Design review of the part built by this model. Coordinates are the model's own, in mm. Give positions to 0.01 mm unless a question says otherwise; leave off trailing zeros. Write each loop counter-clockwise with the first axis right and the second up, starting at its lowest first coordinate (ties: lowest second). Pieces come first, ordered by that corner, then holes. Notation, with made-up numbers: (79.5, -23) -> (111.5, -23) arc R21 cw to (111.5, -16) -> close; hole circle Ø8 at (8.25, 52). An arc over 180 degrees is marked (long way). Return JSON: item names as keys, results as strings. Group by question number.
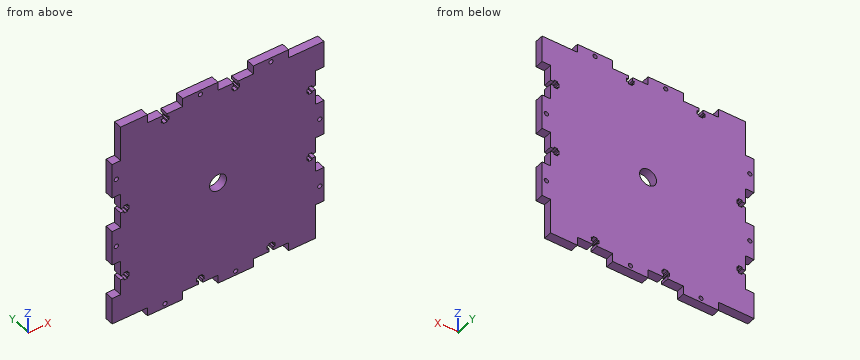
from build123d import *

# Parameters (mm, degrees)
BOSS_EXTRUDE1_DEPTH = 6
SKETCH2_R           = 1.5
CUT_EXTRUDE1_DEPTH  = 107.235587258
SKETCH3_R           = 6
CUT_EXTRUDE2_DEPTH  = 107.235587258


with BuildPart() as part:
    # Sketch1 → Boss-Extrude1 (new body)
    with BuildSketch(Plane(origin=(0, 0, 0), x_dir=(1, 0, 0), z_dir=(0, 1, 0))):
        Polygon((0, 75), (25, 75), (25, 69), (50, 69), (50, 75), (69, 75), (69, 50), (75, 50), (75, 25), (69, 25), (69, 0), (75, 0), (75, -25), (69, -25), (69, -50), (75, -50), (75, -69), (50, -69), (50, -75), (25, -75), (25, -69), (0, -69), (0, -75), (-25, -75), (-25, -69), (-50, -69), (-50, -75), (-69, -75), (-69, -50), (-75, -50), (-75, -25), (-69, -25), (-69, 0), (-75, 0), (-75, 25), (-69, 25), (-69, 50), (-75, 50), (-75, 69), (-50, 69), (-50, 75), (-25, 75), (-25, 69), (0, 69), align=None)
    extrude(amount=BOSS_EXTRUDE1_DEPTH)

    # Sketch2 → Cut-Extrude1 (cut, through all)
    with BuildSketch(Plane(origin=(0, 6, 0), x_dir=(1, 0, 0), z_dir=(0, 1, 0))):
        with Locations(Location((-37.5, 72, 0), (0, 0, 270))):
            Circle(SKETCH2_R)
        with Locations(Location((12.5, 72, 0), (0, 0, 270))):
            Circle(SKETCH2_R)
        with Locations(Location((72, 37.5, 0), (0, 0, 270))):
            Circle(SKETCH2_R)
        with Locations(Location((72, -12.5, 0), (0, 0, 270))):
            Circle(SKETCH2_R)
        with Locations(Location((37.5, -72, 0), (0, 0, 270))):
            Circle(SKETCH2_R)
        with Locations(Location((-12.5, -72, 0), (0, 0, 270))):
            Circle(SKETCH2_R)
        with Locations(Location((-72, -37.5, 0), (0, 0, 270))):
            Circle(SKETCH2_R)
        with Locations(Location((-72, 12.5, 0), (0, 0, 270))):
            Circle(SKETCH2_R)
        with BuildLine():
            Line((-11, 69), (-14, 69))
            Line((-14, 69), (-14, 66.6))
            Line((-14, 66.6), (-15.1, 66.6))
            ThreePointArc((-15.1, 66.6), (-15.270710678, 66.670710678), (-15.2, 66.5))
            Line((-15.2, 66.5), (-15.2, 64.3))
            ThreePointArc((-15.2, 64.3), (-15.270710678, 64.129289322), (-15.1, 64.2))
            Line((-15.1, 64.2), (-14, 64.2))
            Line((-14, 64.2), (-14, 63))
            Line((-14, 63), (-11, 63))
            Line((-11, 63), (-11, 64.2))
            Line((-11, 64.2), (-9.9, 64.2))
            ThreePointArc((-9.9, 64.2), (-9.729289322, 64.129289322), (-9.8, 64.3))
            Line((-9.8, 64.3), (-9.8, 66.5))
            ThreePointArc((-9.8, 66.5), (-9.729289322, 66.670710678), (-9.9, 66.6))
            Line((-9.9, 66.6), (-11, 66.6))
            Line((-11, 66.6), (-11, 69))
        make_face()
        with BuildLine():
            Line((69, 11), (69, 14))
            Line((69, 14), (66.6, 14))
            Line((66.6, 14), (66.6, 15.1))
            ThreePointArc((66.6, 15.1), (66.670710678, 15.270710678), (66.5, 15.2))
            Line((66.5, 15.2), (64.3, 15.2))
            ThreePointArc((64.3, 15.2), (64.129289322, 15.270710678), (64.2, 15.1))
            Line((64.2, 15.1), (64.2, 14))
            Line((64.2, 14), (63, 14))
            Line((63, 14), (63, 11))
            Line((63, 11), (64.2, 11))
            Line((64.2, 11), (64.2, 9.9))
            ThreePointArc((64.2, 9.9), (64.129289322, 9.729289322), (64.3, 9.8))
            Line((64.3, 9.8), (66.5, 9.8))
            ThreePointArc((66.5, 9.8), (66.670710678, 9.729289322), (66.6, 9.9))
            Line((66.6, 9.9), (66.6, 11))
            Line((66.6, 11), (69, 11))
        make_face()
        with BuildLine():
            Line((39, 69), (36, 69))
            Line((36, 69), (36, 66.6))
            Line((36, 66.6), (34.9, 66.6))
            ThreePointArc((34.9, 66.6), (34.729289322, 66.670710678), (34.8, 66.5))
            Line((34.8, 66.5), (34.8, 64.3))
            ThreePointArc((34.8, 64.3), (34.729289322, 64.129289322), (34.9, 64.2))
            Line((34.9, 64.2), (36, 64.2))
            Line((36, 64.2), (36, 63))
            Line((36, 63), (39, 63))
            Line((39, 63), (39, 64.2))
            Line((39, 64.2), (40.1, 64.2))
            ThreePointArc((40.1, 64.2), (40.270710678, 64.129289322), (40.2, 64.3))
            Line((40.2, 64.3), (40.2, 66.5))
            ThreePointArc((40.2, 66.5), (40.270710678, 66.670710678), (40.1, 66.6))
            Line((40.1, 66.6), (39, 66.6))
            Line((39, 66.6), (39, 69))
        make_face()
        with BuildLine():
            Line((69, -39), (69, -36))
            Line((69, -36), (66.6, -36))
            Line((66.6, -36), (66.6, -34.9))
            ThreePointArc((66.6, -34.9), (66.670710678, -34.729289322), (66.5, -34.8))
            Line((66.5, -34.8), (64.3, -34.8))
            ThreePointArc((64.3, -34.8), (64.129289322, -34.729289322), (64.2, -34.9))
            Line((64.2, -34.9), (64.2, -36))
            Line((64.2, -36), (63, -36))
            Line((63, -36), (63, -39))
            Line((63, -39), (64.2, -39))
            Line((64.2, -39), (64.2, -40.1))
            ThreePointArc((64.2, -40.1), (64.129289322, -40.270710678), (64.3, -40.2))
            Line((64.3, -40.2), (66.5, -40.2))
            ThreePointArc((66.5, -40.2), (66.670710678, -40.270710678), (66.6, -40.1))
            Line((66.6, -40.1), (66.6, -39))
            Line((66.6, -39), (69, -39))
        make_face()
        with BuildLine():
            Line((11, -69), (14, -69))
            Line((14, -69), (14, -66.6))
            Line((14, -66.6), (15.1, -66.6))
            ThreePointArc((15.1, -66.6), (15.270710678, -66.670710678), (15.2, -66.5))
            Line((15.2, -66.5), (15.2, -64.3))
            ThreePointArc((15.2, -64.3), (15.270710678, -64.129289322), (15.1, -64.2))
            Line((15.1, -64.2), (14, -64.2))
            Line((14, -64.2), (14, -63))
            Line((14, -63), (11, -63))
            Line((11, -63), (11, -64.2))
            Line((11, -64.2), (9.9, -64.2))
            ThreePointArc((9.9, -64.2), (9.729289322, -64.129289322), (9.8, -64.3))
            Line((9.8, -64.3), (9.8, -66.5))
            ThreePointArc((9.8, -66.5), (9.729289322, -66.670710678), (9.9, -66.6))
            Line((9.9, -66.6), (11, -66.6))
            Line((11, -66.6), (11, -69))
        make_face()
        with BuildLine():
            Line((-39, -69), (-36, -69))
            Line((-36, -69), (-36, -66.6))
            Line((-36, -66.6), (-34.9, -66.6))
            ThreePointArc((-34.9, -66.6), (-34.729289322, -66.670710678), (-34.8, -66.5))
            Line((-34.8, -66.5), (-34.8, -64.3))
            ThreePointArc((-34.8, -64.3), (-34.729289322, -64.129289322), (-34.9, -64.2))
            Line((-34.9, -64.2), (-36, -64.2))
            Line((-36, -64.2), (-36, -63))
            Line((-36, -63), (-39, -63))
            Line((-39, -63), (-39, -64.2))
            Line((-39, -64.2), (-40.1, -64.2))
            ThreePointArc((-40.1, -64.2), (-40.270710678, -64.129289322), (-40.2, -64.3))
            Line((-40.2, -64.3), (-40.2, -66.5))
            ThreePointArc((-40.2, -66.5), (-40.270710678, -66.670710678), (-40.1, -66.6))
            Line((-40.1, -66.6), (-39, -66.6))
            Line((-39, -66.6), (-39, -69))
        make_face()
        with BuildLine():
            Line((-69, 39), (-69, 36))
            Line((-69, 36), (-66.6, 36))
            Line((-66.6, 36), (-66.6, 34.9))
            ThreePointArc((-66.6, 34.9), (-66.670710678, 34.729289322), (-66.5, 34.8))
            Line((-66.5, 34.8), (-64.3, 34.8))
            ThreePointArc((-64.3, 34.8), (-64.129289322, 34.729289322), (-64.2, 34.9))
            Line((-64.2, 34.9), (-64.2, 36))
            Line((-64.2, 36), (-63, 36))
            Line((-63, 36), (-63, 39))
            Line((-63, 39), (-64.2, 39))
            Line((-64.2, 39), (-64.2, 40.1))
            ThreePointArc((-64.2, 40.1), (-64.129289322, 40.270710678), (-64.3, 40.2))
            Line((-64.3, 40.2), (-66.5, 40.2))
            ThreePointArc((-66.5, 40.2), (-66.670710678, 40.270710678), (-66.6, 40.1))
            Line((-66.6, 40.1), (-66.6, 39))
            Line((-66.6, 39), (-69, 39))
        make_face()
        with BuildLine():
            Line((-69, -11), (-69, -14))
            Line((-69, -14), (-66.6, -14))
            Line((-66.6, -14), (-66.6, -15.1))
            ThreePointArc((-66.6, -15.1), (-66.670710678, -15.270710678), (-66.5, -15.2))
            Line((-66.5, -15.2), (-64.3, -15.2))
            ThreePointArc((-64.3, -15.2), (-64.129289322, -15.270710678), (-64.2, -15.1))
            Line((-64.2, -15.1), (-64.2, -14))
            Line((-64.2, -14), (-63, -14))
            Line((-63, -14), (-63, -11))
            Line((-63, -11), (-64.2, -11))
            Line((-64.2, -11), (-64.2, -9.9))
            ThreePointArc((-64.2, -9.9), (-64.129289322, -9.729289322), (-64.3, -9.8))
            Line((-64.3, -9.8), (-66.5, -9.8))
            ThreePointArc((-66.5, -9.8), (-66.670710678, -9.729289322), (-66.6, -9.9))
            Line((-66.6, -9.9), (-66.6, -11))
            Line((-66.6, -11), (-69, -11))
        make_face()
    extrude(amount=-CUT_EXTRUDE1_DEPTH, mode=Mode.SUBTRACT)

    # Sketch3 → Cut-Extrude2 (cut, through all)
    with BuildSketch(Plane.XZ):
        with Locations(Location((0, 0, 0), (0, 0, 270))):
            Circle(SKETCH3_R)
    extrude(amount=-CUT_EXTRUDE2_DEPTH, mode=Mode.SUBTRACT)


solid = part.part
Q1. For L1, parallel to Z at x = 68, y = 2.4; L2, parallel to Z at x = 72, y = 2.4; L3, parallel to Z at x = -72, y = 2.1, list the stretches that pass through material, from the lowest coordinate up. Write a range as from..to.
Q2. Take a section at B-B, the plane y = 4.85. Count the separate pieces of the cut face and the enclosed holes in it, plus the area to 3 significant figures.
Q3. Insertion check: pin 1 (0.9 mm diameter, centred on x = 14.5, y = 3.5, fed in from +Z); pin 2 (0.6 mm diameter, centred on y = 3.5, z = 35.5, fed in from +X); pin 3 (0.6 mm diameter, centred on y = 3.5, z = -39.5, fed in from -X). Each pin has a flat end and moves straight along its axis. Give the tip position at first contact, or say it passes through.
Q4. Take a section at A-A, the plane z = -19. Give the boundary of the cut face in (x, y).
Q5. Take a section at C-C, the plane x = -8. Give the boundary of the cut face in (y, z).
Final values:
{
 "1": {"L1": "z = -75..-14, -11..36, 39..69", "L2": "z = -50..-39, -36..-25, 0..11, 14..25, 50..69", "L3": "z = -69..-50, -25..-14, -11..0, 25..36, 39..50"},
 "2": {"separate pieces": "1", "enclosed holes": "9", "area": "20,300 mm²"},
 "3": {"pin 1": "stops at z = 69", "pin 2": "stops at x = 69", "pin 3": "stops at x = -69"},
 "4": {"outline": "(-75, 0) -> (69, 0) -> (69, 6) -> (-75, 6) -> close"},
 "5": {"outline": "(0, -69) -> (6, -69) -> (6, 75) -> (0, 75) -> close"}
}
